Part model, mm, in its own coordinate system. Face numbers are marked on the shaded views. Round coordinates to 2 decimals unless told otherwise and drop trailing zeros. Loops run counter-clockwise (first coordinate to the right, second up) from the corner with the lowest first, then second, coordinate; pieces in that order, holes last.
1) Mould opens along Y. For the marked faces 1, 2 and 3 say: +Y half, -Y half, draft (parallel to the pull), parting line (faces both ways), or undercut.
2) Band-saw the part on A-A, the plane x = 0. Write the cut outline in (y, z), then the cut area to 3 significant figures.
3) Drop flat-ended pins along their axis: P1, Ø12, axis at x = 2, y = -4.5, coming from the +Z side; P2, Ø3, axis at x = -7, z = -5, coming from the -Y side; P3, Ø3, axis at y = -1.5, z = -3.5, coming from the +X side. Give the stop position or say it passes through.
4) Probe line 1 (Y direction, x = 0, z = -6); line 2 (X direction, y = -4, z = -4.25); line 3 (Z direction, x = 8, y = 13). List the from-to ranges inside material, lowest first.
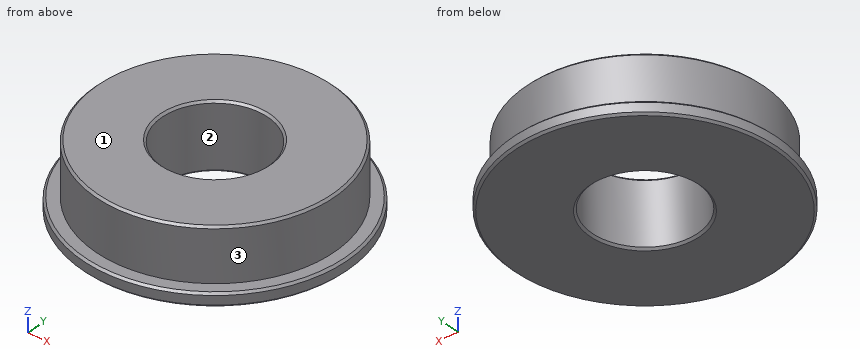
from build123d import *

# Parameters (mm, degrees)
CHAMFER1_SIZE = 0.25


with BuildPart() as part:
    # Sketch1 → Revolve1 (revolve)
    with BuildSketch(Plane(origin=(0, 0, 0), x_dir=(1, 0, 0), z_dir=(0, 1, 0))):
        Polygon((-14.287497289, 6.362699291), (-14.287497289, 0), (-6.349997937, 0), (-6.349997937, 7.937499291), (-15.868754486, 7.937499291), (-15.868754486, 6.362699291), align=None)
    revolve(axis=Axis((0, 0, 0), (0, 0, -1)))

    # Chamfer1
    chamfer1_edges = [part.edges().sort_by_distance(p)[0] for p in [
        (14.287497289, 0, 0),
        (6.349997937, 0, 0),
        (6.349997937, 0, -7.937499291),
        (15.868754486, 0, -7.937499291),
        (15.868754486, 0, -6.362699291),
    ]]
    chamfer(chamfer1_edges, length=CHAMFER1_SIZE)


solid = part.part
Reported:
1. face 1: draft
1. face 2: undercut
1. face 3: parting line
2. outline: (-15.87, -7.69) - (-15.62, -7.94) - (-6.6, -7.94) - (-6.35, -7.69) - (-6.35, -0.25) - (-6.6, 0) - (-14.04, 0) - (-14.29, -0.25) - (-14.29, -6.36) - (-15.62, -6.36) - (-15.87, -6.61) - close; (6.35, -7.69) - (6.6, -7.94) - (15.62, -7.94) - (15.87, -7.69) - (15.87, -6.61) - (15.62, -6.36) - (14.29, -6.36) - (14.29, -0.25) - (14.04, 0) - (6.6, 0) - (6.35, -0.25) - close
2. area: 131 mm2
3. P1: stops at z = 0
3. P2: stops at y = -14.26
3. P3: stops at x = 14.29
4. line 1: y = -14.29 to -6.35, 6.35 to 14.29
4. line 2: x = -13.72 to -4.93, 4.93 to 13.72
4. line 3: z = -7.94 to -6.36
